Verification items for the finished model (mm, model axes). A direction names the side the tool comes from. Give positions to 0.01 mm unless a question says otherwise; leave off trailing zeros. Order: outer loops, then holes, each group sorted by start corner. A loop starts at its lowest first (then second) coordinate and runs counter-clockwise, first axis right, second up. Notation, with made-up numbers: (53, 12.25) -> (57, 12.25) arc R26 cw to (57, 42.25) -> close; hole circle Ø9 at (-20, 84.5). An arc over 180 degrees is marked (long way). Return JSON: item names as keys, results as strings. Group by question number.
(1) Cross-section at B-B on y = 18. Enter the section's corners in (x, z), then the cut area to 3 significant figures.
(2) Depth check by flat-ended pin: pin 1 Ø8 at (x, z) = (228.5, -260.5) entering from +Y. Enter the tip coordinate at first touch or a pass-through.
(3) Thickness scan on line 1 along X through (y, z) = (61.5, -97); line 2 along X through (y, z) = (74, -231); line 3 along Z through (x, y) = (133.5, 26.5). Record the ranges inside material, lowest first.
(4) Cross-section at A-A on z = -353.5. Enter the section's corners in (x, y), then the cut area to 3 significant figures.
(5) Release check for a two-part mould opening along Z. For faces 4 (the face through (68.03, 37.567, -390.303)), 5 (the face through (206, 44, -419.1)), 6 (the face through (206, 44, -38.1)), 7 (the face through (406, 114.3, -76)) record: pulls with the +Z half, pulls with the -Z half, needs draft (parallel to the pull), parting line crosses it, or undercut.
(6) Cross-section at C-C on x = 106. Enter the section's corners in (y, z), then the cut area to 3 significant figures.
(7) Tool access check on faces 1 (the face through (0, 44, -226)), 2 (the face through (385, 38, -406.4)), 3 (the face through (38.112, 101.422, -75.642)). Record the directions out of +Z, -Z, +X, -X, +Y, -Y that give a thin tool (end or side, any length) a straight path to the whole face; none if there is none.
(8) Cross-section at D-D on y = 106.5. Enter the section's corners in (x, z), then the cut area to 3 significant figures.
Autodesk Inventor part; units mm, degrees
ref_plane "YZ Plane" through (0, 0, 0) normal (1, 0, 0) x (0, 1, 0)
ref_plane "XZ Plane" through (0, 0, 0) normal (0, 1, 0) x (-1, 0, 0)
ref_plane "XY Plane" through (0, 0, 0) normal (0, 0, 1) x (1, 0, 0)
sketch "Sketch1" plane through (0, 0, 0) normal (0, 1, 0) x (-1, 0, 0)
  line L0 (0, 0) -> (-457.2, 0) construction
  line L1 (-457.2, -457.2) -> (0, -457.2) construction
  line L2 (0, -457.2) -> (0, 0) construction
  line L3 (0, 0) -> (0, -38.1) construction
  line L4 (0, -457.2) -> (0, -419.1) construction
  line L5 (0, -38.1) -> (0, -371.3712)
  line L6 (-457.2, -76.2) -> (-457.2, -381)
  line L7 (0, -371.3712) -> (0, -419.1)
  line L8 (-406.4, -38.1) -> (-457.2, -76.2)
  line L9 (-406.4, -419.1) -> (-457.2, -381)
  line L10 (-457.2, 0) -> (-457.2, -38.1) construction
  line L11 (-457.2, -76.2) -> (-457.2, -457.2) construction
  line L12 (-444.5, -82.55) -> (-444.5, -374.65)
  line L13 (-444.5, -374.65) -> (-402.1667, -406.4)
  line L14 (-12.7, -406.4) -> (-12.7, -371.3712)
  line L15 (-12.7, -371.3712) -> (-12.7, -50.8)
  line L16 (-402.1667, -50.8) -> (-444.5, -82.55)
  line L17 (-444.5, -82.55) -> (-444.5, -374.65)
  line L18 (-444.5, -374.65) -> (-402.1667, -406.4)
  line L19 (-12.7, -406.4) -> (-12.7, -371.3712)
  line L20 (-12.7, -371.3712) -> (-12.7, -50.8)
  line L21 (-402.1667, -50.8) -> (-444.5, -82.55)
  line L22 (-444.5, -82.55) -> (-444.5, -374.65)
  line L23 (-12.7, -406.4) -> (-12.7, -50.8)
  line L24 (-444.5, -82.55) -> (-444.5, -374.65)
  line L25 (-402.1667, -50.8) -> (-12.7, -50.8)
  line L26 (-406.4, -38.1) -> (0, -38.1)
  line L27 (-406.4, -419.1) -> (0, -419.1)
  line L28 (-402.1667, -406.4) -> (-12.7, -406.4)
  dimension "d0" = 457.2
  dimension "d1" = 457.2
  dimension "d12" = 12.7
  dimension "d13" = 12.7
extrude "Extrusion1" add sketch "Sketch1" along normal blind 88.9 contours L5 L7 L27 L9 L6 L8 L26 | L16 L25 L15 L14 L28 L13 L12
sketch "Sketch2" plane through (0, 0, 0) normal (0, -1, 0) x (1, 0, 0)
  line L0 (0, -38.1) -> (0, -419.1)
  line L1 (406.4, -419.1) -> (457.2, -381)
  line L2 (457.2, -381) -> (457.2, -76.2)
  line L3 (457.2, -76.2) -> (406.4, -38.1)
  line L4 (402.1667, -50.8) -> (444.5, -82.55)
  line L5 (444.5, -82.55) -> (444.5, -374.65)
  line L6 (444.5, -374.65) -> (402.1667, -406.4)
  line L7 (402.1667, -406.4) -> (368.3, -406.4)
  line L8 (368.3, -406.4) -> (368.3, -330.2)
  line L9 (368.3, -330.2) -> (88.9, -330.2)
  line L10 (88.9, -330.2) -> (88.9, -374.65)
  line L11 (88.9, -374.65) -> (46.5667, -406.4)
  line L12 (46.5667, -406.4) -> (12.7, -406.4)
  line L13 (12.7, -406.4) -> (12.7, -50.8)
  line L14 (12.7, -50.8) -> (46.5667, -50.8)
  line L15 (46.5667, -50.8) -> (88.9, -82.55)
  line L16 (88.9, -82.55) -> (88.9, -127)
  line L17 (88.9, -127) -> (368.3, -127)
  line L18 (368.3, -127) -> (368.3, -50.8)
  line L19 (368.3, -50.8) -> (402.1667, -50.8)
  line L20 (0, -419.1) -> (406.4, -419.1)
  line L21 (406.4, -38.1) -> (0, -38.1)
  point P0 (0, 0)
  dimension "d14" = 12.7
extrude "Extrusion2" cut sketch "Sketch2" against normal blind 76.2 contours L4 L5 L6 L7 L8 L9 L10 L11 L12 L13 L14 L15 L16 L17 L18 L19
sketch "Sketch3" plane through (0, 88.9, 0) normal (0, 1, 0) x (1, 0, 0)
  line L0 (0, 419.1) -> (0, 38.1)
  line L1 (406.4, 38.1) -> (457.2, 76.2)
  line L2 (457.2, 76.2) -> (457.2, 381)
  line L3 (457.2, 381) -> (406.4, 419.1)
  circle A0 centre (50.8, 76.2) radius 12.7
  circle A1 centre (50.8, 381) radius 12.7
  circle A2 centre (406.4, 381) radius 12.7
  circle A3 centre (406.4, 76.2) radius 12.7
  line L4 (0, 38.1) -> (406.4, 38.1)
  line L5 (406.4, 419.1) -> (0, 419.1)
  point P0 (0, 0)
  dimension "d17" = 25.4
  dimension "d18" = 25.4
  dimension "d19" = 25.4
  dimension "d20" = 25.4
extrude "Extrusion3" add sketch "Sketch3" along normal blind 25.4 contours A0 | A1 | A2 | A3
properties part number "Body Base" material "Aluminum 6061"
Verdict:
{
 "1": {"outline": "(0, -419.1) -> (406.4, -419.1) -> (457.2, -381) -> (457.2, -76.2) -> (406.4, -38.1) -> (0, -38.1) -> close; hole (12.7, -406.4) -> (46.57, -406.4) -> (88.9, -374.65) -> (88.9, -330.2) -> (368.3, -330.2) -> (368.3, -406.4) -> (402.17, -406.4) -> (444.5, -374.65) -> (444.5, -82.55) -> (402.17, -50.8) -> (368.3, -50.8) -> (368.3, -127) -> (88.9, -127) -> (88.9, -82.55) -> (46.57, -50.8) -> (12.7, -50.8) -> close", "area": "64,000 mm²"},
 "2": {"pin 1": "y = 88.9"},
 "3": {"line 1": "0 to 12.7, 88.9 to 368.3, 444.5 to 457.2", "line 2": "0 to 12.7, 444.5 to 457.2", "line 3": "-419.1 to -330.2, -127 to -38.1"},
 "4": {"outline": "(0, 0) -> (12.7, 0) -> (12.7, 76.2) -> (88.9, 76.2) -> (88.9, 0) -> (368.3, 0) -> (368.3, 76.2) -> (444.5, 76.2) -> (444.5, 0) -> (457.2, 0) -> (457.2, 88.9) -> (0, 88.9) -> close", "area": "29,000 mm²"},
 "5": {"face 4": "undercut", "face 5": "pulls with the -Z half", "face 6": "pulls with the +Z half", "face 7": "needs draft"},
 "6": {"outline": "(0, -419.1) -> (88.9, -419.1) -> (88.9, -38.1) -> (0, -38.1) -> (0, -127) -> (76.2, -127) -> (76.2, -330.2) -> (0, -330.2) -> close", "area": "18,400 mm²"},
 "7": {"face 1": "+Z, -Z, -X, +Y, -Y", "face 2": "-Y", "face 3": "+Y"},
 "8": {"outline": "circle Ø25.4 at (50.8, -381); circle Ø25.4 at (50.8, -76.2); circle Ø25.4 at (406.4, -381); circle Ø25.4 at (406.4, -76.2)", "area": "2,030 mm²"}
}
